The listing builds one solid part. Answer for the finished solid, in the listing's coordinates (mm). Face numbers are marked on the shaded views. A direction names the side the tool comes from. Coordinates: 2 decimals unless noted, no trailing zeros. Order: outer loops, then holes, each group sorted by start corner. A loop starts at its lowest first (then second) coordinate and runs counter-clockwise, first axis right, second up. Notation, with made-up numbers: M 81.25,31.25 L 118.25,31.25 A25 cw 118.25,55.25 Z; hole C -40,-1.75 d11. An arc over 180 degrees is marked long. One line per item, written item: value. Start each with the question number.
Q1. For the marked faces 1 and 2, determine the directions among +Z, -Z, +X, -X, +Y, -Y from which every point of the face is accessible in a straight line to the end or side of a thin tool.
Q2. The part is cut by section C-C on z = -6.5. Give the vertices of the cut face in (x, y).
Q3. Straight lines are drawn through the part: line 1 along Y through (x, z) = (0, -5); line 2 along Z through (x, y) = (-4, 2.5); line 3 along Z through (x, y) = (-2.75, 1.25). For each, find the intervals that lie inside material, in ascending order. Write a range as [from, to].
Q4. The part is cut by section A-A on y = 0. Give the vertices of the cut face in (x, z), then the cut area to 4 significant figures.
Q5. The part is cut by section D-D on z = 1. Give the vertices of the cut face in (x, y).
Q6. Each of these flat-tipped pins is pushed along its axis until it touches: pin 1 Ø1 at (y, z) = (2, 2) entering from +X; pin 2 Ø5 at (y, z) = (3, -5.5) entering from -X; pin 3 Ø3 at (y, z) = (0.5, 10) entering from -X. Where does it stop, or does it pass through?
Q7. Determine the mould class of the marked faces 3, 4 and 5 for opening direction Y: pulls with the +Y half, pulls with the -Y half, needs draft (parallel to the pull), parting line crosses it, or undercut.
Autodesk Fusion 360 part; units mm, degrees
sketch "Sketch1" plane through (0, 0, 0) normal (0, 0, 1) x (1, 0, 0)
  circle A0 centre (0, 0) radius 2.85
  circle A1 centre (0, 0) radius 5
  dimension "d1" = 5.7
  dimension "d2" = 10
extrude "Extrude1" add sketch "Sketch1" along normal blind 13 contours A0
ref_plane "WorkPlane1" through (0, 0, -11) normal (0, 0, 1) x (1, 0, 0)
sketch "Sketch2" plane through (0, 0, -11) normal (0, 0, 1) x (1, 0, 0)
  circle A0 centre (0, 0) radius 5
  circle A1 centre (0, 0) radius 3.1
  dimension "d6" = 10
  dimension "d7" = 6.2
extrude "Extrude2" add sketch "Sketch2" along normal blind 11 contours A0 | A1
extrude "Extrude3" cut sketch "Sketch2" along normal blind 8 contours A1
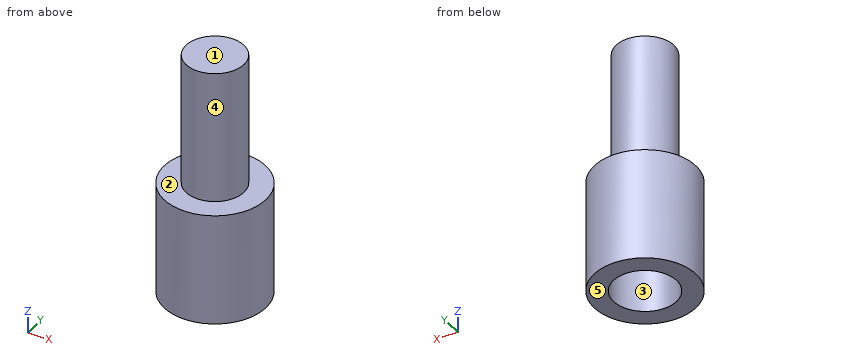
Output:
1. face 1: +Z, +X, -X, +Y, -Y
1. face 2: +Z
2. outline: C 0,0 d10; hole C 0,0 d6.2
3. line 1: y = [-5, -3.1], [3.1, 5]
3. line 2: z = [-11, 0]
3. line 3: z = [-3, 0]
4. outline: M -5,-11 L -3.1,-11 L -3.1,-3 L 3.1,-3 L 3.1,-11 L 5,-11 L 5,0 L 2.85,0 L 2.85,13 L -2.85,13 L -2.85,0 L -5,0 Z
4. area: 134.5 mm^2
5. outline: C 0,0 d5.7
6. pin 1: stops at x = 2.42
6. pin 2: stops at x = -4.97
6. pin 3: stops at x = -2.85
7. face 3: undercut
7. face 4: parting line crosses it
7. face 5: needs draft
